from build123d import *

# Parameters (mm, degrees)
BOSS_EXTRUDE1_DEPTH = 17
SKETCH4_R           = 1.6
CUT_EXTRUDE2_DEPTH  = 1


with BuildPart() as part:
    # Sketch1 → Boss-Extrude1 (new body)
    with BuildSketch(Plane(origin=(0, 0, 0), x_dir=(1, 0, 0), z_dir=(0, 1, 0))):
        with BuildLine():
            Line((1.322591209, -4.028579324), (4.779691323, -4.028579324))
            Line((4.779691323, -4.028579324), (4.779691323, -1.028579324))
            Line((4.779691323, -1.028579324), (3.051141266, -1.028579324))
            Line((3.051141266, -1.028579324), (-0.984859984, 2.26705444))
            ThreePointArc((-0.984859984, 2.26705444), (-1.156228622, 3.119019075), (-1.325410362, 3.971420676))
            Line((-1.325410362, 3.971420676), (-4.382631249, 3.971420676))
            ThreePointArc((-4.382631249, 3.971420676), (-3.983741211, 1.961503644), (-3.572803177, -0.045984755))
            ThreePointArc((-3.572803177, -0.045984755), (-1.83279885, -2.907176181), (1.322591209, -4.028579324))
        make_face()
        with BuildLine():
            Line((3.779691323, -3.028579324), (3.779691323, -2.028579324))
            Line((3.779691323, -2.028579324), (2.694726151, -2.028579324))
            Line((2.694726151, -2.028579324), (-1.893840411, 1.718256703))
            ThreePointArc((-1.893840411, 1.718256703), (-2.020759818, 2.344719816), (-2.146500023, 2.971420676))
            Line((-2.146500023, 2.971420676), (-3.166177568, 2.971420676))
            ThreePointArc((-3.166177568, 2.971420676), (-2.882916081, 1.563855286), (-2.5937243, 0.157496332))
            ThreePointArc((-2.5937243, 0.157496332), (-1.201720839, -2.131456809), (1.322591209, -3.028579324))
            Line((1.322591209, -3.028579324), (3.779691323, -3.028579324))
        make_face(mode=Mode.SUBTRACT)
    extrude(amount=BOSS_EXTRUDE1_DEPTH)

    # Sketch4 → Cut-Extrude2 (cut)
    with BuildSketch(Plane(origin=(0.716662117, 0, -0.877660993), x_dir=(-0.774572925, 0, -0.632484612), z_dir=(0.632484612, 0, -0.774572925))):
        with Locations((-0.408584542, 8.5)):
            Circle(SKETCH4_R)
    extrude(amount=-CUT_EXTRUDE2_DEPTH, mode=Mode.SUBTRACT)


solid = part.part
Read the model definition and answer for the solid it produces. Units are mm, in the model's axes. A direction names the side the tool comes from. Give positions to 0.01 mm unless a question says otherwise; leave off trailing zeros. Write each loop counter-clockwise with the first axis right and the second up, starting at its lowest first coordinate (ties: lowest second). Pieces come first, ordered by that corner, then holes. Notation, with made-up numbers: M 3.25,58.25 L 54.25,58.25 A8 ccw 54.25,62.25 Z; hole C 54,-16.75 d3. An arc over 180 degrees is marked long. One line per item, written item: value. Start each with the question number.
(1) Find section C-C (z = 2.25). Determine the outline of the cut face in (x, y).
(2) A tool of negligible diameter and unlimited length cuts with its end or side. For faces 4 (the cylindrical face through (-1.23, 8.38, 2.11)), 5 (the flat face through (-3, 8, -3.971)), 6 (the flat face through (4, 8, 1.029)), from which of +Z, -Z, +X, -X, +Y, -Y can it reach the whole face along a straight path? Write none if from no direction.
(3) Find section B-B (y = 13). Determine the outline of the cut face in (x, z).
(4) Find section D-D (y = 8). Determine the outline of the cut face in (x, z), plus the area to 3 significant figures.
(5) Find section A-A (x = 3.5). Determine the outline of the cut face in (y, z), plus the area to 3 significant figures.
(6) Determine the mould class of faces 1 (the flat face through (4.78, 8, 3)), 2 (the flat face through (3, 8, 4.029)), 3 (the flat face through (3.78, 8.4, 2.5)) for opening direction Z: pulls with the +Z half, pulls with the -Z half, needs draft (parallel to the pull), parting line crosses it, or undercut.
(7) Flat-ended cylindrical pins translate along their axes: pin 1 Ø3 at (y, z) = (15, -2) entering from +X; pin 2 Ø3 at (x, y) = (4, 10) entering from -Z; pin 3 Ø1.4 at (x, y) = (4, 12.5) entering from -Z. Find the tip coordinate at first contact, or state that the pin passes through.
(8) Find the intervals of material crossed by line 1 (Z direction, x = 1.25, y = 7.75); line 2 (X direction, y = 14.75, z = -1); line 3 (X direction, y = 12.5, z = -2), in increasing order.
Results below:
1. outline: M -2.5,0 L -1.05,0 L -1.05,17 L -2.5,17 Z; M 3.78,0 L 4.78,0 L 4.78,17 L 3.78,17 Z
2. face 4: +Y, -Y
2. face 5: -Z, +X, -X, +Y, -Y
2. face 6: -Z, +X, +Y, -Y
3. outline: M -4.38,-3.97 L -1.33,-3.97 A338.64 cw -0.98,-2.27 L 3.05,1.03 L 4.78,1.03 L 4.78,4.03 L 1.32,4.03 A5 ccw -3.57,0.05 A341.64 ccw Z; hole M -3.17,-2.97 L -2.15,-2.97 A339.64 cw -1.89,-1.72 L 2.69,2.03 L 3.78,2.03 L 3.78,3.03 L 1.32,3.03 A4 ccw -2.59,-0.16 A340.64 ccw Z
4. outline: M -4.38,-3.97 L -1.33,-3.97 A338.64 cw -0.98,-2.27 L -0.14,-1.58 L -0.78,-0.81 L -1.89,-1.72 A339.64 ccw -2.15,-2.97 L -3.17,-2.97 A340.64 cw -2.59,-0.16 A4 cw 1.32,3.03 L 3.78,3.03 L 3.78,2.03 L 2.69,2.03 L 1.58,1.12 L 2.21,0.34 L 3.05,1.03 L 4.78,1.03 L 4.78,4.03 L 1.32,4.03 A5 ccw -3.57,0.05 A341.64 ccw Z
4. area: 22.1 mm^2
5. outline: M 0,1.03 L 17,1.03 L 17,2.03 L 0,2.03 Z; M 0,3.03 L 17,3.03 L 17,4.03 L 0,4.03 Z
5. area: 34.0 mm^2
6. face 1: needs draft
6. face 2: pulls with the +Z half
6. face 3: undercut
7. pin 1: stops at x = 1.18
7. pin 2: stops at z = 0.58
7. pin 3: stops at z = 1.03
8. line 1: z = 3.03 to 4.03
8. line 2: x = -3.79 to -2.77, -1.01 to 0.57
8. line 3: x = -3.99 to -2.97, -1.95 to -0.66
